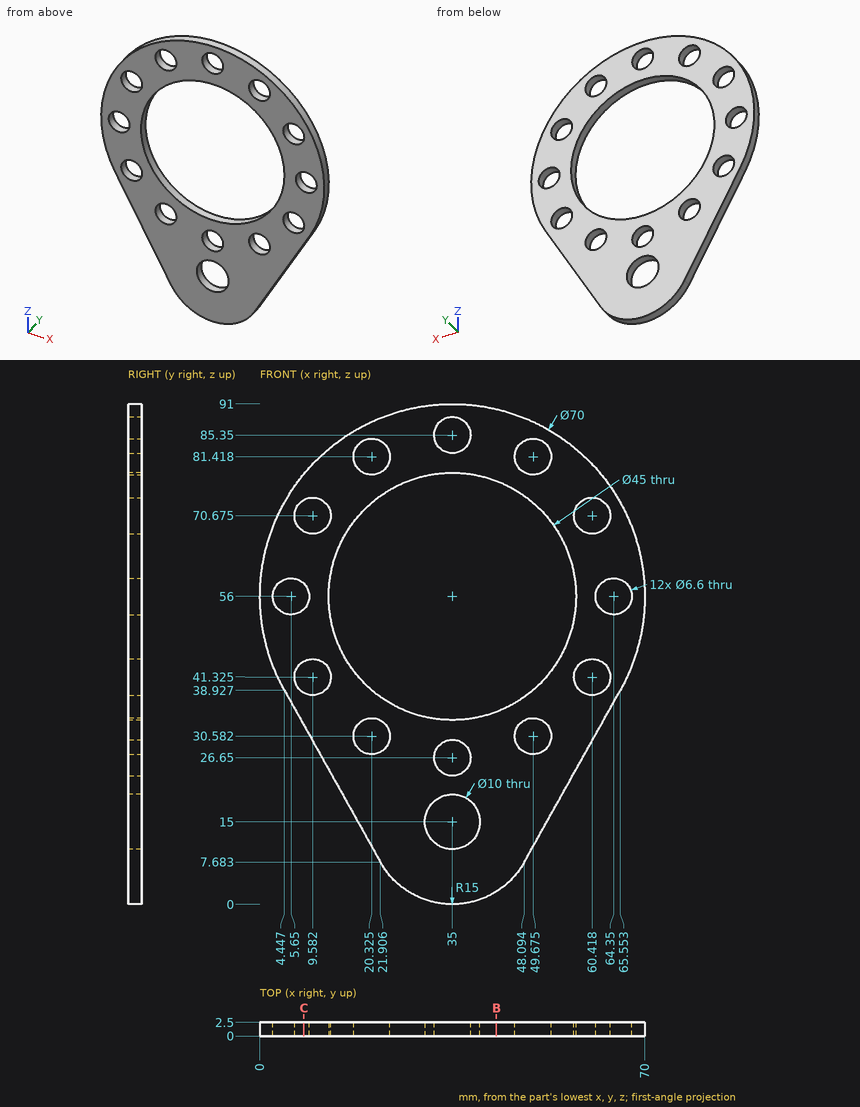
The figure shows three views and two pictorial views of one solid part (mm, origin at its lowest corner). Answer the questions. Round coordinates to 2 decimals unless told otherwise and drop trailing zeros. Loops run counter-clockwise (first coordinate to the right, second up) from the corner with the lowest first, then second, coordinate; pieces in that order, holes last. Notation, with made-up numbers: (87.5, 81) - (131.5, 81) arc R28 ccw to (131.5, 108) - close; hole circle Ø10 at (-39.5, 22.5). An arc over 180 degrees is marked (long way). One line per question, with ' | ' between items. Start each with the question number.
Q1. Find the intervals of material crossed by L1, parallel to Z at x = 61, y = 0.5 (1 decimal); L2, parallel to Z at x = 33, y = 1.75 (1 decimal); L3, parallel to X at y = 0.7, z = 57.5, in increasing order.
Q2. Section C-C on x = 8 is taken. Give the vertices of the cut face in (y, z).
Q3. A flat-ended cylindrical pin translates along its axis: pin 1 (7.5 mm diameter, centred on x = 9.58, z = 70.68, fed in from -Y). Find the tip coordinate at first contact, or state that the pin passes through.
Q4. Section B-B on x = 43 is taken. Give the vertices of the cut face in (y, z), plus the area to 3 significant figures.
Established:
1) L1: 30.8 to 38.1, 44.6 to 67.4, 73.9 to 79.4 | L2: 0.1 to 10.4, 19.6 to 24, 29.3 to 33.6, 78.4 to 82.7, 88 to 90.9 | L3: 0.03 to 2.71, 8.59 to 12.55, 57.45 to 61.41, 67.29 to 69.97
2) outline: (0, 32.57) - (2.5, 32.57) - (2.5, 38.43) - (0, 38.43) - close; (0, 44.22) - (2.5, 44.22) - (2.5, 53.68) - (0, 53.68) - close; (0, 58.32) - (2.5, 58.32) - (2.5, 67.78) - (0, 67.78) - close; (0, 73.57) - (2.5, 73.57) - (2.5, 78.27) - (0, 78.27) - close
3) pin 1: y = 0
4) outline: (0, 2.31) - (2.5, 2.31) - (2.5, 34.97) - (0, 34.97) - close; (0, 77.03) - (2.5, 77.03) - (2.5, 90.07) - (0, 90.07) - close | area: 114 mm²
